Geometry: final body of the model. Coordinates: model frame, mm. Give positions to 0.01 mm unless a question says otherwise; leave off trailing zeros. Loops run counter-clockwise (first coordinate to the right, second up) from the corner with the lowest first, then second, coordinate; pieces in that order, holes last.
1. Section C-C, the plane z = 3.5. Output: boundary loops of the cut face in (x, y), then the cut area to 3 significant figures.
2. First-contact query: P1, Ø0.5, axis at y = 1.5, z = 4, coming from the -X side. Flat tip, straight axial feed; report the tip coordinate or a pass-through.
3. Material intervals for line 1 along X through (y, z) = (0, 2.5); line 2 along Y through (x, z) = (0, 4.75); line 3 along X through (y, z) = (0.65, 6), sorted ascending.
4. Section B-B, the plane x = 0.9. Output: boundary loops of the cut face in (y, z).
5. Section A-A, the plane y = 0. Output: boundary loops of the cut face in (x, z), then the cut area to 3 significant figures.
6. Draft query along X for faces 1 (the face through (0.74, 1.526, 7.131)), 2 (the face through (-1.526, -0.017, 7.131)), 3 (the face through (0.05, -1.15, 3.94)). Return one class per face: +X half, -X half, draft (parallel to the pull), parting line (faces both ways), or undercut.
7. Section D-D, the plane x = 0. Output: boundary loops of the cut face in (y, z), then the cut area to 3 significant figures.
Autodesk Inventor part; units mm, degrees
ref_plane "YZ Plane" through (0, 0, 0) normal (1, 0, 0) x (0, 1, 0)
ref_plane "XZ Plane" through (0, 0, 0) normal (0, 1, 0) x (-1, 0, 0)
ref_plane "XY Plane" through (0, 0, 0) normal (0, 0, 1) x (1, 0, 0)
sketch "Sketch1" plane through (0, 0, 0) normal (0, 0, 1) x (1, 0, 0)
  line L0 (-1.2, 1.6) -> (-0.2919, 1.6)
  line L1 (1.6, 1.2) -> (1.6, -1.2)
  line L2 (1.2, -1.6) -> (-1.2, -1.6)
  line L3 (-1.6, -1.2) -> (-1.6, 1.2)
  line L4 (0, -2.356) -> (0, 2.356)
  line L5 (-2.356, 0) -> (2.356, 0)
  arc A0 (-0.2919, 1.1123) -> (0.2919, 1.1123) centre (0, 0) ccw
  line L6 (0.2919, 1.6) -> (0.2919, 1.1123)
  line L7 (0.2919, 1.6) -> (1.2, 1.6)
  line L8 (-0.2919, 1.1123) -> (-0.2919, 1.6)
  arc A1 (1.6, 1.2) -> (1.2, 1.6) centre (1.2, 1.2) ccw
  arc A2 (1.2, -1.6) -> (1.6, -1.2) centre (1.2, -1.2) ccw
  arc A3 (-1.6, -1.2) -> (-1.2, -1.6) centre (-1.2, -1.2) ccw
  arc A4 (-1.2, 1.6) -> (-1.6, 1.2) centre (-1.2, 1.2) ccw
  dimension "d0" = 1.6
  dimension "d2" = 2.3
  dimension "d6" = 0.4
extrude "Extrusion2" add sketch "Sketch1" along normal blind 8 contours L0 L8 A0 L5 L3 A4 | L5 A0 L4 L2 A3 L3 | A0 L5 L1 A2 L2 L4 | A0 L6 L7 A1 L1 L5
chamfer "Chamfer1" distance 0.15 angle 85 9 edges at (1.6, 0, 8) (1.4828, 1.4828, 8) (0.746, 1.6, 8) (1.4828, -1.4828, 8) (0, -1.6, 8) (-1.4828, -1.4828, 8) (-1.6, 0, 8) (-1.4828, 1.4828, 8) (-0.746, 1.6, 8) measured on face at (-1.4476, 0.0429, 8)
equation "\"d0\" = d1"
properties part number "hjul-motor overgang"
Answers below:
1. outline: (-1.6, -1.2) arc R0.4 ccw to (-1.2, -1.6) - (1.2, -1.6) arc R0.4 ccw to (1.6, -1.2) - (1.6, 1.2) arc R0.4 ccw to (1.2, 1.6) - (0.29, 1.6) - (0.29, 1.11) arc R1.15 cw (long way) to (-0.29, 1.11) - (-0.29, 1.6) - (-1.2, 1.6) arc R0.4 ccw to (-1.6, 1.2) - close
1. area: 5.68 mm2
2. P1: stops at x = -1.6
3. line 1: x = -1.6 to -1.15, 1.15 to 1.6
3. line 2: y = -1.6 to -1.15
3. line 3: x = -1.6 to -0.95, 0.95 to 1.6
4. outline: (-1.6, 0) - (-0.72, 0) - (-0.72, 8) - (-1.45, 8) - (-1.6, 6.29) - close; (0.72, 0) - (1.6, 0) - (1.6, 6.29) - (1.45, 8) - (0.72, 8) - close
5. outline: (-1.6, 0) - (-1.15, 0) - (-1.15, 8) - (-1.45, 8) - (-1.6, 6.29) - close; (1.15, 0) - (1.6, 0) - (1.6, 6.29) - (1.45, 8) - (1.15, 8) - close
5. area: 6.94 mm2
6. face 1: draft
6. face 2: -X half
6. face 3: undercut
7. outline: (-1.6, 0) - (-1.15, 0) - (-1.15, 8) - (-1.45, 8) - (-1.6, 6.29) - close
7. area: 3.47 mm2
